For this review, take the finished solid that the model builds, in its own axes (mm). A direction names the side the tool comes from. Round coordinates to 2 decimals unless told otherwise and drop trailing zeros. Write each loop counter-clockwise with the first axis right and the second up, starting at its lowest first coordinate (ties: lowest second). Pieces come first, ordered by that corner, then holes. Notation, with made-up numbers: M 70,-9 L 94,-9 A8 cw 94,-4 Z; hole C -21,24.25 d7. An arc over 180 degrees is marked long. Write each question's results on one line, items separated by ' | '. Start each with the question number.
Solid Edge part; units mm, degrees
sketch "Sketch1" plane through (0, 0, 0) normal (0, -1, 0) x (1, 0, 0)
  line L0 (20.5, 17.5) -> (20.5, -17.5)
  line L1 (20.5, -17.5) -> (-20.5, -17.5)
  line L2 (-20.5, -17.5) -> (-20.5, 17.5)
  line L3 (-20.5, 17.5) -> (20.5, 17.5)
  dimension "D1" = 20.5
  dimension "D2" = 20.5
extrude "Protrusion1" add sketch "Sketch1" along normal mid plane 19.5
sketch "Sketch2" plane through (17.7914, 0, 17.5) normal (0, 0, 1) x (1, 0, 0)
  line L0 (-24.6483, 8.939) -> (-4.2914, 8.939)
  line L1 (-4.2914, 8.939) -> (-4.2914, 5)
  line L2 (-4.2914, -5) -> (-4.2914, -8.939)
  line L3 (-4.2914, -8.939) -> (-24.6483, -8.939)
  arc A0 (-24.6483, -8.939) -> (-24.6483, 8.939) centre (-28.5414, 0) cw
  arc A1 (-4.2914, 5) -> (-4.2914, -5) centre (-4.2914, 0) cw
  dimension "D1" = 4.2914
extrude "ProtrusiónExtruida_3" add sketch "Sketch2" along normal blind 1
sketch "Sketch3" plane through (16.3242, 0, 18.5) normal (0, 0, 1) x (1, 0, 0)
  circle A0 centre (-26.3242, 0) radius 6.5
extrude "ProtrusiónExtruida_4" add sketch "Sketch3" along normal blind 2
sketch "Sketch4" plane through (7.7914, 0, 20.5) normal (0, 0, 1) x (1, 0, 0)
  circle A0 centre (-17.7914, 0) radius 3
extrude "ProtrusiónExtruida_5" add sketch "Sketch4" along normal blind 4
sketch "Sketch5" plane through (-20.5, 0, 10.2776) normal (-1, 0, 0) x (0, 0, 1)
  line L0 (-24.2776, 3.75) -> (-24.2776, -3.75)
  line L1 (-20.2776, -3.75) -> (-24.2776, -3.75)
  line L2 (-20.2776, 3.75) -> (-20.2776, -3.75)
  line L3 (-24.2776, 3.75) -> (-20.2776, 3.75)
  dimension "D1" = 24.2776
  dimension "D2" = 24.2776
  dimension "D3" = 24.2776
extrude "ProtrusiónExtruida_6" add sketch "Sketch5" along normal blind 2
Item 1: We need section D-D on z = -3. State the section outline as (x, y) points.
Item 2: We need section A-A on x = 9. State the section outline as (y, z) points, then the cut area to 3 significant figures.
Item 3: For faces 1 (the flat face through (-21, 0, -10)), 2 (the flat face through (-21, 0, -14)), 3 (the cylindrical face through (-20.496, -0.27, 17.993)), 4 (the flat face through (-21, 3.75, -12)), list the 3-axis set-ups (+Z, -Z, +X, -X, +Y, -Y) from which the entire face can be reached by the end or side of a thin tool; tool diameter is ignored.
Item 4: We need section B-B on z = -12. State the section outline as (x, y) points.
Item 5: We need section C-C on x = -8.5. State the section outline as (y, z) points, then the cut area to 3 significant figures.
Item 6: Insertion check: P1, Ø6, axis at x = 5.5, y = -2.5, coming from the +Z side; P2, Ø4, axis at y = 4, z = -7, coming from the -X side; P3, Ø0.8, axis at y = 7, z = 18, coming from the +X side. Each pin has a flat end and moves straight along its axis. Give the tip position at first contact, or say it passes through.
Item 7: For probe 1 along Z at (x, y) = (-4.5, -2.5); probe 2 along Z at (x, y) = (1.5, -8.5); probe 3 along X at (y, z) = (-3.25, 11), list the stretches that pass through material, from the lowest coordinate up.
Numbers:
1) outline: M -20.5,-9.75 L 20.5,-9.75 L 20.5,9.75 L -20.5,9.75 Z
2) outline: M -9.75,-17.5 L 9.75,-17.5 L 9.75,17.5 L 8.94,17.5 L 8.94,18.5 L -8.94,18.5 L -8.94,17.5 L -9.75,17.5 Z | area: 700 mm^2
3) face 1: +Z, -X, +Y, -Y | face 2: -Z, -X, +Y, -Y | face 3: +Z | face 4: +Z, -Z, -X, +Y
4) outline: M -22.5,-3.75 L -20.5,-3.75 L -20.5,-9.75 L 20.5,-9.75 L 20.5,9.75 L -20.5,9.75 L -20.5,3.75 L -22.5,3.75 Z
5) outline: M -9.75,-17.5 L 9.75,-17.5 L 9.75,17.5 L 9.49,17.5 L 9.49,18.5 L 6.32,18.5 L 6.32,20.5 L 2.6,20.5 L 2.6,24.5 L -2.6,24.5 L -2.6,20.5 L -6.32,20.5 L -6.32,18.5 L -9.49,18.5 L -9.49,17.5 L -9.75,17.5 Z | area: 748 mm^2
6) P1: stops at z = 18.5 | P2: stops at x = -20.5 | P3: stops at x = 13.5
7) probe 1: z = -17.5 to 20.5 | probe 2: z = -17.5 to 18.5 | probe 3: x = -20.5 to 20.5
